The model under review builds one solid part; all positions refer to its coordinate system, in mm. A direction names the side the tool comes from. Round coordinates to 2 decimals unless told otherwise and drop trailing zeros. Loops run counter-clockwise (first coordinate to the right, second up) from the corner with the lowest first, then second, coordinate; pieces in that order, holes last. Notation, with made-up numbers: M 58,15 L 85,15 A15 cw 85,44 Z; hole C 60.5,-23 d7. An arc over 180 degrees is marked long. Answer as a JSON object with one key per item and string values. Group by question number.
Item 1: Insertion check: P1, Ø1.5, axis at y = 2, z = 22, coming from the +X side; P2, Ø3, axis at y = 8.5, z = 82.5, coming from the -X side; P3, Ø22, axis at x = 0, z = 0, coming from the -Y side; P4, Ø5, axis at x = 20.5, y = 4, coming from the -Z side. Each pin has a flat end and moves straight along its axis. Give the tip position at first contact, or say it passes through.
Item 2: Tool access review of faces 1 (the face through (-56.158, 5, 65)), 2 (the face through (-2.646, 5.634, 11.914)): name each direction out of +Z, -Z, +X, -X, +Y, -Y from which nothing blocks a thin tool from reaching the whole face with its end or side.
Item 3: Consider section C-C (z = 22.5). Give the boundary of the cut face in (x, y), and give its area (3 significant figures).
Item 4: Consider section B-B (y = 5). Give the boundary of the cut face in (x, z), and give its area (3 significant figures).
Item 5: Consider section D-D (x = 25). Give the boundary of the cut face in (y, z), and give its area (3 significant figures).
Item 6: Consider section A-A (x = 6.5). Give the boundary of the cut face in (y, z), and give its area (3 significant figures).
Item 7: The part is to be moulded in two halves that separate along Y. For faces 3 (the face through (43.9, 5.478, -44.853)), 4 (the face through (-1, 0, 32)), 5 (the face through (-1, 11.112, 32)), say which applies: +Y half, -Y half, draft (parallel to the pull), parting line (faces both ways), or undercut.
Item 8: To check wall thickness, follow line 1 (Z direction, x = 0, y = 8.5); line 2 (Z direction, x = 16, y = 6.5); line 3 (Z direction, x = -34, y = 9.25). State the ranges of each line that lie inside material, in increasing order.
```python
from build123d import *

# Parameters (mm, degrees)
SKETCH1_R           = 7.9375
BOSS_EXTRUDE1_DEPTH = 11.1125
SKETCH2_R           = 12.20390625
CUT_EXTRUDE1_DEPTH  = 11.1125


with BuildPart() as part:
    # Sketch1 → Boss-Extrude1 (new body)
    with BuildSketch(Plane(origin=(0, 0, 0), x_dir=(1, 0, 0), z_dir=(0, 1, 0))):
        with BuildLine():
            Line((-56.1578125, 0), (-56.1578125, -131.7625))
            Line((-56.1578125, -131.7625), (37.9015625, -131.7625))
            ThreePointArc((37.9015625, -131.7625), (40.48606485, -64.852857695), (57.15, 0))
            ThreePointArc((57.15, 0), (43.44844613, 45.367716005), (0, 64.29375))
            ThreePointArc((0, 64.29375), (-44.848953518, 46.794786657), (-56.1578125, 0))
        make_face()
        Circle(SKETCH1_R, mode=Mode.SUBTRACT)
    extrude(amount=BOSS_EXTRUDE1_DEPTH)

    # Sketch2 → Cut-Extrude1 (cut)
    with BuildSketch(Plane(origin=(0, 11.1125, 0), x_dir=(1, 0, 0), z_dir=(0, 1, 0))):
        Circle(SKETCH2_R)
    extrude(amount=-CUT_EXTRUDE1_DEPTH, mode=Mode.SUBTRACT)


solid = part.part
```
Geometry results:
{
 "1": {"P1": "stops at x = 50.05", "P2": "stops at x = -56.16", "P3": "passes through", "P4": "stops at z = -61.77"},
 "2": {"face 1": "+Z, -X, +Y, -Y", "face 2": "+Y, -Y"},
 "3": {"outline": "M -56.16,0 L 49.69,0 L 49.69,11.11 L -56.16,11.11 Z", "area": "1,180 mm^2"},
 "4": {"outline": "M -56.16,0 A52.04 ccw 0,-64.29 A56.43 ccw 57.15,0 A315.1 cw 37.9,131.76 L -56.16,131.76 Z; hole C 0,0 d24.41", "area": "18,700 mm^2"},
 "5": {"outline": "M 0,-59.08 L 11.11,-59.08 L 11.11,131.76 L 0,131.76 Z", "area": "2,120 mm^2"},
 "6": {"outline": "M 0,-64.07 L 11.11,-64.07 L 11.11,-10.33 L 0,-10.33 Z; M 0,10.33 L 11.11,10.33 L 11.11,131.76 L 0,131.76 Z", "area": "1,950 mm^2"},
 "7": {"face 3": "draft", "face 4": "-Y half", "face 5": "+Y half"},
 "8": {"line 1": "z = -64.29 to -12.2, 12.2 to 131.76", "line 2": "z = -62.35 to 131.76", "line 3": "z = -56.2 to 131.76"}
}
